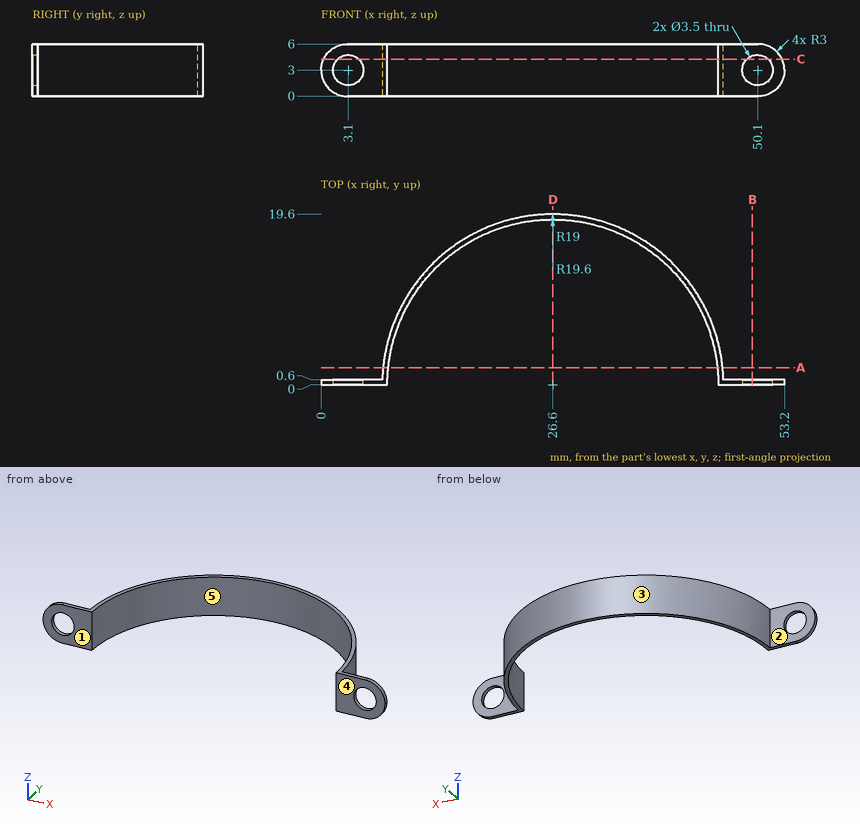
The drawing under review shows one solid part. Ordinate dimensions are in mm from its lowest x, y, z. A direction names the side the tool comes from. Coordinates: 2 decimals unless noted, no trailing zeros. Order: outer loops, then holes, each group sorted by start corner. A loop starts at its lowest first (then second) coordinate and runs counter-clockwise, first axis right, second up. Notation, with made-up numbers: (-10.5, 58.25) -> (7.5, 58.25) arc R19 ccw to (7.5, 83.25) -> close; hole circle Ø10 at (35.5, 6.25). An arc over 180 degrees is marked (long way). Answer in a Markdown table with one row per item. Add a question column.
Item 1: We need section B-B on x = 49.5. Write out the cut boundary in (y, z).
Item 2: Clearance check with flat-ended pins moving along their axes: pin 1 (10 mm diameter, centred on x = 13.5, y = 7.5, fed in from -Z); pin 2 (1.8 mm diameter, centred on x = 2, z = 2, fed in from +Y); pin 3 (3 mm diameter, centred on y = 12.5, z = 2, fed in from -X); pin 4 (10 mm diameter, centred on x = 7.5, y = 16.5, fed in from -Z). State where each tip first meets the part, or that it passes through.
Item 3: To check wall thickness, follow probe 1 along Z at (x, y) = (3.1, 0.4); probe 2 along Y at (x, z) = (26.5, 3); probe 3 along X at (y, z) = (4.25, 4.75). State the ranges of each line that lie inside material, in increasing order.
Item 4: Mouldability with a two-part tool opening along X and no side actions: class the marked faces 3, 4 and 5 as +X half, -X half, draft (parallel to the pull), parting line (faces both ways), or undercut.
Item 5: Machinability: for the marked faces 1 and 2, which of the approach directions +Z, -Z, +X, -X, +Y, -Y give a long, thin tool a straight path to every point of the face, cutting with its end or side? Answer none if there is none.
Item 6: We need section C-C on z = 4.25. Write out the cut boundary in (x, y), plus the area to 3 significant figures.
Item 7: We need section A-A on y = 2. Write out the cut boundary in (x, z).
Item 8: We need section D-D on x = 26.6. Write out the cut boundary in (y, z).
Final values:
| question | item | result |
|---|---|---|
| 1 | outline | (0, 0) -> (0.6, 0) -> (0.6, 1.36) -> (0, 1.36) -> close; (0, 4.64) -> (0.6, 4.64) -> (0.6, 6) -> (0, 6) -> close |
| 2 | pin 1 | stops at z = 0 |
| 2 | pin 2 | stops at y = 0.6 |
| 2 | pin 3 | stops at x = 10.38 |
| 2 | pin 4 | passes through |
| 3 | probe 1 | z = 0 to 1.25, 4.75 to 6 |
| 3 | probe 2 | y = 19 to 19.6 |
| 3 | probe 3 | x = 7.47 to 8.08, 45.12 to 45.73 |
| 4 | face 3 | parting line |
| 4 | face 4 | draft |
| 4 | face 5 | undercut |
| 5 | face 1 | +Z, -Z, +X, -X, -Y |
| 5 | face 2 | +Z, -Z, -X, +Y |
| 6 | outline | (0.27, 0) -> (1.88, 0) -> (1.88, 0.6) -> (0.27, 0.6) -> close; (4.32, 0) -> (7.6, 0) arc R19 cw to (45.6, 0) -> (48.88, 0) -> (48.88, 0.6) -> (46.19, 0.6) arc R19.6 ccw to (7.01, 0.6) -> (4.32, 0.6) -> close; (51.32, 0) -> (52.93, 0) -> (52.93, 0.6) -> (51.32, 0.6) -> close |
| 6 | area | 41.5 mm2 |
| 7 | outline | (7.1, 0) -> (7.71, 0) -> (7.71, 6) -> (7.1, 6) -> close; (45.49, 0) -> (46.1, 0) -> (46.1, 6) -> (45.49, 6) -> close |
| 8 | outline | (19, 0) -> (19.6, 0) -> (19.6, 6) -> (19, 6) -> close |
